Autodesk Inventor part; units mm, degrees
ref_plane "YZ Plane" through (0, 0, 0) normal (1, 0, 0) x (0, 1, 0)
ref_plane "XZ Plane" through (0, 0, 0) normal (0, 1, 0) x (-1, 0, 0)
ref_plane "XY Plane" through (0, 0, 0) normal (0, 0, 1) x (1, 0, 0)
sketch "Sketch1" plane through (0, 0, 0) normal (1, 0, 0) x (0, 1, 0)
  line L0 (0, 0) -> (0, -36)
  line L1 (0, 0) -> (36, 0) construction
  line L2 (0, 0) -> (147, 0)
  line L3 (147, 0) -> (147, -36)
  line L4 (147, -36) -> (0, -36)
  line L5 (147, -36) -> (147, -39)
  line L6 (147, -39) -> (-3, -39)
  line L7 (-3, -39) -> (-3, 3)
  line L8 (-3, 3) -> (150, 3)
  line L9 (150, 3) -> (150, -39)
  line L10 (150, -39) -> (147, -39)
  dimension "d0" = 36
  dimension "d1" = 90
  dimension "d2" = 147
  dimension "d3" = 3
  dimension "d4" = 150
  dimension "d5" = 42
  dimension "d6" = 153
extrude "Extrusion1" add sketch "Sketch1" along normal blind 54
sketch "Sketch2" plane through (54, 0, 0) normal (1, 0, 0) x (0, 0, -1)
  line L0 (39, 150) -> (-3, 150)
  line L1 (-3, 150) -> (-3, -3)
  line L2 (-3, -3) -> (39, -3)
  line L3 (39, -3) -> (39, 150)
  line L4 (36, 147) -> (36, 0)
  line L5 (36, 0) -> (0, 0)
  line L6 (0, 0) -> (0, 147)
  line L7 (0, 147) -> (36, 147)
extrude "Extrusion2" add sketch "Sketch2" along normal blind 4 contours L3 L2 L1 L0 | L4 L5 L6 L7
sketch "Sketch3" plane through (0, -3, -39) normal (0, -1, 0) x (1, 0, 0)
  line L0 (0, 42) -> (0, 0)
  line L1 (0, 0) -> (58, 0)
  line L2 (58, 42) -> (58, 0)
  line L3 (0, 42) -> (58, 42)
  line L4 (0, 0) -> (0, 42)
  line L5 (0, 42) -> (0, 39)
  line L6 (0, 3) -> (0, 39)
  line L7 (0, 39) -> (10, 39)
  line L8 (0, 39) -> (54, 39)
  line L9 (0, 39) -> (10, 39) construction
  line L10 (10, 39) -> (10, 3)
  line L11 (10, 3) -> (0, 3)
  line L12 (0, 3) -> (0, 0)
  dimension "d11" = 10
  dimension "d12" = 0
  dimension "d13" = 36
extrude "Extrusion3" cut sketch "Sketch3" against normal blind 4 contours L7 L10 L11 L0
sketch "Sketch4" plane through (58, 0, 0) normal (1, 0, 0) x (0, 0, -1)
  line L0 (-3, 150) -> (-3, -3)
  line L1 (-3, -3) -> (39, -3)
  line L2 (39, -3) -> (39, 150)
  line L3 (39, 150) -> (-3, 150)
  line L4 (-3, 150) -> (-3, -3)
  line L5 (-3, -3) -> (-3, 32)
  line L6 (-3, 150) -> (-3, 115)
  line L7 (-3, 115) -> (-3, 111)
  line L8 (-3, 111) -> (39, 111)
  line L9 (39, -3) -> (39, 150)
  line L10 (39, 111) -> (39, 115)
  line L11 (39, 115) -> (-3, 115)
  line L12 (-3, 32) -> (-3, 36)
  line L13 (-3, 36) -> (39, 36)
  line L14 (39, 36) -> (39, 32)
  line L15 (39, 32) -> (-3, 32)
  point P0 (0, 0)
  dimension "d16" = 35
  dimension "d17" = 35
  dimension "d18" = 4
  dimension "d19" = 4
  dimension "d20" = 4
extrude "Extrusion4" cut sketch "Sketch4" against normal blind 2 contours L11 L2 L8 L0 | L13 L2 L15 L0
fillet "Fillet1" radius 2 12 edges at (29, 150, 3) (58, 132.5, 3) (58, 73.5, 3) (58, 150, -18) (58, 132.5, -39) (58, 73.5, -39) (58, 14.5, -39) (58, 14.5, 3) (29, -3, 3) (58, -3, -18) (29, -3, -39) (29, 150, -39)
properties part number "carcasa_lippo"
For this review, take the finished solid that the model builds, in its own axes (mm). A direction names the side the tool comes from. Give positions to 0.01 mm unless a question says otherwise; leave off trailing zeros. Write each loop counter-clockwise with the first axis right and the second up, starting at its lowest first coordinate (ties: lowest second). Pieces come first, ordered by that corner, then holes. Notation, with made-up numbers: M 16.25,34 L 66.25,34 A20 ccw 66.25,45 Z; hole C -2.5,47.5 d2. An arc over 180 degrees is marked long. Answer as a JSON object with one key per item and string values. Group by question number.
Item 1: Consider section B-B on y = 69.5. Write out the cut boundary in (x, z), plus the area to 3 significant figures.
Item 2: Consider section A-A on x = 37. Write out the cut boundary in (y, z), plus the area to 3 significant figures.
Item 3: Draft analysis for pull direction Z (two halves, no side actions). For faces 4 (the flat face through (28, 72, 3)), 5 (the flat face through (54, 75, -18)), 6 (the flat face through (58, 74, -18)), 7 (the flat face through (10, -2, -18)), state which applies: +Z half, -Z half, draft (parallel to the pull), parting line (faces both ways), or undercut.
Item 4: For probe 1 along Y at (x, z) = (22.5, -30); probe 2 along Z at (x, y) = (26, 68); probe 3 along X at (y, z) = (13, -5), list the stretches that pass through material, from the lowest coordinate up. Write a range as [from, to].
Item 5: For pin 1 Ø3 at (y, z) = (105.5, -9.5) entering from -X; pin 2 Ø1.6 at (x, z) = (57.5, -28) entering from -Y; pin 3 Ø0.6 at (x, z) = (56.5, -22.5) entering from -Y, all flat-tipped, find the tip position at first contact; note any pin that passes through.
Item 6: Consider section C-C on z = -3.5. Write out the cut boundary in (x, y), plus the area to 3 significant figures.
Item 7: Tool access review of faces 1 (the flat face through (34, -3, -18)), 2 (the flat face through (32, 0, -18)), 3 (the flat face through (56, 113, -18)): name each direction out of +Z, -Z, +X, -X, +Y, -Y from which nothing blocks a thin tool from reaching the whole face with its end or side.
Check result:
{
 "1": {"outline": "M 0,-39 L 56,-39 A2 ccw 58,-37 L 58,1 A2 ccw 56,3 L 0,3 L 0,0 L 54,0 L 54,-36 L 0,-36 Z", "area": "490 mm^2"},
 "2": {"outline": "M -3,-37 A2 ccw -1,-39 L 148,-39 A2 ccw 150,-37 L 150,1 A2 ccw 148,3 L -1,3 A2 ccw -3,1 Z; hole M 0,-36 L 147,-36 L 147,0 L 0,0 Z", "area": "1,130 mm^2"},
 "3": {"face 4": "+Z half", "face 5": "undercut", "face 6": "draft", "face 7": "undercut"},
 "4": {"probe 1": "y = [-3, 0], [147, 150]", "probe 2": "z = [-39, -36], [0, 3]", "probe 3": "x = [54, 58]"},
 "5": {"pin 1": "stops at x = 54", "pin 2": "stops at y = -2.87", "pin 3": "stops at y = -2.99"},
 "6": {"outline": "M 0,147 L 54,147 L 54,0 L 10,0 L 10,-3 L 56,-3 A2 ccw 58,-1 L 58,32 L 56,32 L 56,36 L 58,36 L 58,111 L 56,111 L 56,115 L 58,115 L 58,148 A2 ccw 56,150 L 0,150 Z", "area": "888 mm^2"},
 "7": {"face 1": "+Z, -Z, +X, -X, -Y", "face 2": "-X", "face 3": "+Z, -Z, +X"}
}
